Here's how the part is built. I have some questions about the finished solid (model axes, mm). A direction names the side the tool comes from. Give positions to 0.01 mm unless a question says otherwise; leave off trailing zeros. Write each loop counter-clockwise with the first axis right and the second up, starting at its lowest first coordinate (ties: lowest second). Pieces come first, ordered by that corner, then holes. Notation, with made-up numbers: (-18, -7.5) -> (39, -7.5) arc R29 ccw to (39, 31.5) -> close; hole circle Ø2 at (-6, 35). An arc over 180 degrees is marked (long way). Return JSON: item names as keys, results as strings.
from build123d import *

# Parameters (mm, degrees)
BOSS_EXTRUDE3_DEPTH = 3.9
SKETCH2_R           = 2.4
CUT_EXTRUDE1_DEPTH  = 7.8
SKETCH3_R           = 3.05
CUT_EXTRUDE2_DEPTH  = 0.8
SKETCH4_R           = 3.05
CUT_EXTRUDE3_DEPTH  = 0.8


with BuildPart() as part:
    # Sketch1 → Boss-Extrude3 (new body)
    with BuildSketch(Plane(origin=(0, 0, 0), x_dir=(1, 0, 0), z_dir=(0, 1, 0))):
        with BuildLine():
            Line((-16, -3.7), (24, -3.7))
            ThreePointArc((24, -3.7), (27.7, 0), (24, 3.7))
            Line((24, 3.7), (-16, 3.7))
            ThreePointArc((-16, 3.7), (-19.7, 0), (-16, -3.7))
        make_face()
    extrude(amount=BOSS_EXTRUDE3_DEPTH)

    # Sketch2 → Cut-Extrude1 (cut)
    with BuildSketch(Plane(origin=(0, 3.9, 0), x_dir=(1, 0, 0), z_dir=(0, 1, 0))):
        Circle(SKETCH2_R)
        with Locations((8, 0)):
            Circle(SKETCH2_R)
        with Locations((16, 0)):
            Circle(SKETCH2_R)
        with Locations((-16, 0)):
            Circle(SKETCH2_R)
        with Locations((-8, 0)):
            Circle(SKETCH2_R)
        with Locations((24, 0)):
            Circle(SKETCH2_R)
    extrude(amount=-CUT_EXTRUDE1_DEPTH, mode=Mode.SUBTRACT)

    # Sketch3 → Cut-Extrude2 (cut)
    with BuildSketch(Plane(origin=(0, 3.9, 0), x_dir=(1, 0, 0), z_dir=(0, 1, 0))):
        Circle(SKETCH3_R)
        with Locations((8, 0)):
            Circle(SKETCH3_R)
        with Locations((16, 0)):
            Circle(SKETCH3_R)
        with Locations((-16, 0)):
            Circle(SKETCH3_R)
        with Locations((-8, 0)):
            Circle(SKETCH3_R)
        with Locations((24, 0)):
            Circle(SKETCH3_R)
    extrude(amount=-CUT_EXTRUDE2_DEPTH, mode=Mode.SUBTRACT)

    # Sketch4 → Cut-Extrude3 (cut)
    with BuildSketch(Plane.XZ):
        Circle(SKETCH4_R)
        with Locations((8, 0)):
            Circle(SKETCH4_R)
        with Locations((16, 0)):
            Circle(SKETCH4_R)
        with Locations((-16, 0)):
            Circle(SKETCH4_R)
        with Locations((-8, 0)):
            Circle(SKETCH4_R)
        with Locations((24, 0)):
            Circle(SKETCH4_R)
    extrude(amount=-CUT_EXTRUDE3_DEPTH, mode=Mode.SUBTRACT)


solid = part.part
1. For pin 1 Ø3.5 at (x, z) = (-16, 0) entering from +Y; pin 2 Ø3 at (x, z) = (7, 1) entering from +Y; pin 3 Ø1.5 at (y, z) = (1, 1.5) entering from -X; pin 4 Ø3 at (x, z) = (7, -1) entering from -Y, each with a flat end and sliding along its axis, tell me the tip position at first contact or that it passes through.
Taken from the geometry:
{"pin 1": "passes through", "pin 2": "stops at y = 3.1", "pin 3": "stops at x = -19.62", "pin 4": "stops at y = 0.8"}
2. Suppose I cut it at C-C, the plane z = 0. Count the separate pieces of the cut face and the enclosed holes in it, and give its area (3 significant figures).
Taken from the geometry:
{"separate pieces": "7", "enclosed holes": "0", "area": "60.1 mm²"}
3. If we mould it in two halves opening along Z, with no side actions, what happens to faces 1 (the face through (26.817, 0.394, -1.168)), 2 (the face through (27.7, 1.9, 0.1)), 3 (the face through (4, 2, 3.7))? For each: released by +Z, released by -Z, zero draft, split by the parting line, or undercut.
Taken from the geometry:
{"face 1": "undercut", "face 2": "split by the parting line", "face 3": "released by +Z"}
4. Suppose I cut it at A-A, the plane y = 2.3. List the corners of the cut face in (x, z) for me, and give its area (3 significant figures).
Taken from the geometry:
{"outline": "(-16, -3.7) -> (24, -3.7) arc R3.7 ccw to (24, 3.7) -> (-16, 3.7) arc R3.7 ccw to start; hole circle Ø4.8 at (-16, 0); hole circle Ø4.8 at (-8, 0); hole circle Ø4.8 at (0, 0); hole circle Ø4.8 at (8, 0); hole circle Ø4.8 at (16, 0); hole circle Ø4.8 at (24, 0)", "area": "230 mm²"}
5. If I drill on line 1 (Z direction, x = 0, y = 3.7); line 2 (Z direction, x = -16, y = 1.45); line 3 (Y direction, x = 6, z = 2.25), over which ranges is the centre line in solid material (lowest first)? Write a range as [from, to].
Taken from the geometry:
{"line 1": "z = [-3.7, -3.05], [3.05, 3.7]", "line 2": "z = [-3.7, -2.4], [2.4, 3.7]", "line 3": "y = [0.8, 3.1]"}
6. Which directions (+Z, -Z, +X, -X, +Y, -Y) give clear straight access to the entire face, cutting with the end or side of a thin tool? Please do faces 4 (the face through (-3.047, 3.506, -0.134)), 5 (the face through (26.29, 1.97, -0.72)), 6 (the face through (-11.047, 0.394, 0.134)).
Taken from the geometry:
{"face 4": "+Y", "face 5": "+Y, -Y", "face 6": "-Y"}
7. Suppose I cut it at D-D, the plane x = 15. List the corners of the cut face in (y, z) for me.
Taken from the geometry:
{"outline": "(0, -3.7) -> (3.9, -3.7) -> (3.9, -2.88) -> (3.1, -2.88) -> (3.1, -2.18) -> (0.8, -2.18) -> (0.8, -2.88) -> (0, -2.88) -> close; (0, 2.88) -> (0.8, 2.88) -> (0.8, 2.18) -> (3.1, 2.18) -> (3.1, 2.88) -> (3.9, 2.88) -> (3.9, 3.7) -> (0, 3.7) -> close"}
8. Suppose I cut it at B-B, the plane x = -8. List the corners of the cut face in (y, z) for me.
Taken from the geometry:
{"outline": "(0, -3.7) -> (3.9, -3.7) -> (3.9, -3.05) -> (3.1, -3.05) -> (3.1, -2.4) -> (0.8, -2.4) -> (0.8, -3.05) -> (0, -3.05) -> close; (0, 3.05) -> (0.8, 3.05) -> (0.8, 2.4) -> (3.1, 2.4) -> (3.1, 3.05) -> (3.9, 3.05) -> (3.9, 3.7) -> (0, 3.7) -> close"}
